Check sheet for the modelled part. Datum: model origin and axes. Units: mm. Coordinates: 2 decimals unless noted, no trailing zeros. Return JSON: item names as keys, results as strings.
from build123d import *

# Parameters (mm, degrees)
PATTERN_CIRCULAR_3_COUNT = 4


with BuildPart() as part:
    # 草图1 → 旋转1 (revolve)
    with BuildSketch(Plane(origin=(0, 0, 0), x_dir=(1, 0, 0), z_dir=(0, 1, 0))):
        with BuildLine():
            Line((0, 0), (0, -36.748051116))
            Line((0, -36.748051116), (-7.524654351, -36.748051116))
            add(Edge.make_bspline(
                [(-2.395571036, 0), (-2.395571036, -10.269932721), (-4.281645701, -29.256357428), (-7.524654351, -36.748051116)],
                knots=[0, 0, 0, 0, 1, 1, 1, 1], degree=3))
            Line((-2.395571036, 0), (0, 0))
        make_face()
    revolve_1 = revolve(axis=Axis((0, 0, 0), (0, 0, 1)))

    # 阵列(圆周)3: 旋转1 ×4 about axis
    pattern_circular_3_axis = Axis((0, 5.442530379, 0), (0, -1, 0))
    for i in range(1, PATTERN_CIRCULAR_3_COUNT):
        add(revolve_1.rotate(pattern_circular_3_axis, i * 360 / PATTERN_CIRCULAR_3_COUNT))


solid = part.part
1) Section check A-A on y = -5. Count the separate pieces of the cut face and the enclosed holes in it, then the cut area to 3 significant figures.
Answers:
{"separate pieces": "4", "enclosed holes": "0", "area": "242 mm²"}
2) Scan lines: line 1 along X through (y, z) = (-1, -25); line 2 along Y through (x, z) = (33.5, 0.5); line 3 along X through (y, z) = (-3.5, -24). Record each from-to range of solid material in increasing order. Write a range as [from, to].
Answers:
{"line 1": "[-4.44, 4.44]", "line 2": "[-6.37, 6.37]", "line 3": "[-2.65, 2.65]"}
3) Go/stop test with flat-tipped pins: pin 1 Ø2 at (y, z) = (-1, -9) entering from +X; pin 2 Ø8 at (x, z) = (19.5, 9) entering from -Y; pin 3 Ø8 at (y, z) = (5, 17.5) entering from +X; pin 4 Ø8 at (x, y) = (-18, 4.5) entering from -Z. Record where each tip stops, or that it passes through.
Answers:
{"pin 1": "x = 2.77", "pin 2": "through", "pin 3": "x = 3.46", "pin 4": "z = -3.68"}
